```python
from build123d import *

# Parameters (mm, degrees)
BOSS_EXTRU_1_DEPTH      = 10
ESQUISSE2_W             = 15
ESQUISSE2_H             = 48
BOSS_EXTRU_2_DEPTH      = 250
ESQUISSE5_W             = 230
ESQUISSE5_H             = 48
ENL_V_MAT_EXTRU_1_DEPTH = 15
ESQUISSE6_R             = 5
ENL_V_MAT_EXTRU_2_DEPTH = 250


with BuildPart() as part:
    # Esquisse1 → Boss.-Extru.1 (new body)
    with BuildSketch(Plane(origin=(0, 0, 0), x_dir=(1, 0, 0), z_dir=(0, 1, 0))):
        Polygon((-210, 0), (-250, 0), (-250, 36.228880697), (-211.024769455, 36.228880697), (-211.024769455, 121.442108629), (-250, 121.442108629), (-250, 200), (-211.024769455, 200), (0, 200), (0, 0), align=None)
    extrude(amount=BOSS_EXTRU_1_DEPTH)

    # Esquisse2 → Boss.-Extru.2 (add)
    with BuildSketch(Plane(origin=(0, 0, 0), x_dir=(0, 0, -1), z_dir=(1, 0, 0))):
        with Locations((192.5, 34)):
            Rectangle(ESQUISSE2_W, ESQUISSE2_H)
    extrude(amount=-BOSS_EXTRU_2_DEPTH)

    # Esquisse5 → Enlèv. mat.-Extru.1 (cut)
    with BuildSketch(Plane.XY.offset(-185)):
        with Locations((-125, 34)):
            Rectangle(ESQUISSE5_W, ESQUISSE5_H)
    extrude(amount=-ENL_V_MAT_EXTRU_1_DEPTH, mode=Mode.SUBTRACT)

    # Esquisse6 → Enlèv. mat.-Extru.2 (cut)
    with BuildSketch(Plane(origin=(0, 0, 0), x_dir=(0, 0, -1), z_dir=(1, 0, 0))):
        with Locations((192.5, 50.5)):
            Circle(ESQUISSE6_R)
    extrude(amount=-ENL_V_MAT_EXTRU_2_DEPTH, mode=Mode.SUBTRACT)


solid = part.part
```
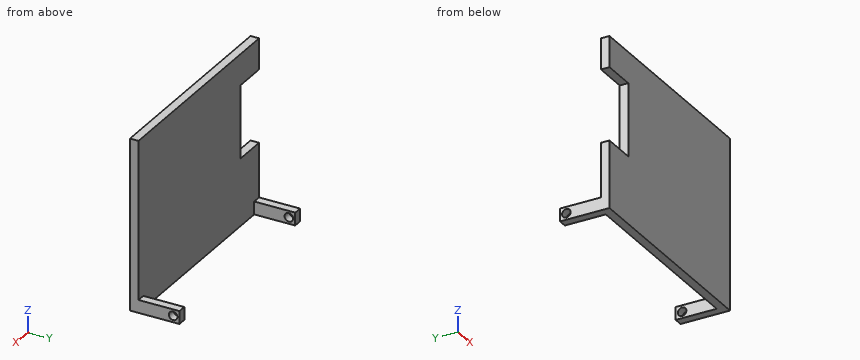
The listing builds one solid part. Answer for the finished solid, in the listing's coordinates (mm). Coordinates: 2 decimals unless noted, no trailing zeros. Loops run counter-clockwise (first coordinate to the right, second up) from the corner with the lowest first, then second, coordinate; pieces in that order, holes last. Notation, with made-up numbers: M 88,69.25 L 100,69.25 A26 ccw 100,94.25 Z; hole C 12,52 d10. An arc over 180 degrees is marked long. Answer as CSV lines item,"result". Start each with the question number.
(1) The part is cut by section B-B (z = -192.5). Give the vertices of the cut face in (x, y).
(2) The part is cut by section D-D (x = -108). Give the vertices of the cut face in (y, z).
(3) The part is cut by section A-A (y = 31.5). Give the vertices of the cut face in (x, z).
(4) The part is cut by section C-C (y = 50.5). Give the vertices of the cut face in (x, z).
(5) Given pin 1 (5 mm diameter, centred on x = -226, y = 7.5, fed in from +Z); pin 2 (5 mm diameter, centred on x = -246, y = 44.5, fed in from +Z); pin 3 (4 mm diameter, centred on y = 13.5, z = -135.5, fed in from +X); pin 4 (2 mm diameter, centred on x = -111, z = -147, fed in from +Y), each flat-ended and moving along its own axis, determine where each tip first touches the part or whether it passes through.
(6) Find the intervals of material crossed by L1, parallel to X at y = 31, z = -188; L2, parallel to Y at x = -5, z = -192; L3, parallel to Z at x = -4, y = 50, in increasing order. Write a range as [from, to].
Determined:
1,outline,"M -250,0 L 0,0 L 0,45.5 L -10,45.5 L -10,10 L -240,10 L -240,45.5 L -250,45.5 Z; M -250,55.5 L -240,55.5 L -240,58 L -250,58 Z; M -10,55.5 L 0,55.5 L 0,58 L -10,58 Z"
2,outline,"M 0,-200 L 10,-200 L 10,0 L 0,0 Z"
3,outline,"M -250,-200 L -240,-200 L -240,-185 L -250,-185 Z; M -10,-200 L 0,-200 L 0,-185 L -10,-185 Z"
4,outline,"M -250,-200 L -240,-200 L -240,-197.5 L -250,-197.5 Z; M -250,-187.5 L -240,-187.5 L -240,-185 L -250,-185 Z; M -10,-200 L 0,-200 L 0,-197.5 L -10,-197.5 Z; M -10,-187.5 L 0,-187.5 L 0,-185 L -10,-185 Z"
5,pin 1,"z = 0"
5,pin 2,"z = -185"
5,pin 3,"through"
5,pin 4,"y = 10"
6,L1,"[-250, -240], [-10, 0]"
6,L2,"[0, 45.53], [55.47, 58]"
6,L3,"[-200, -197.47], [-187.53, -185]"
